Autodesk Inventor part; units mm, degrees
ref_plane "YZ Plane" through (0, 0, 0) normal (1, 0, 0) x (0, 1, 0)
ref_plane "XZ Plane" through (0, 0, 0) normal (0, 1, 0) x (-1, 0, 0)
ref_plane "XY Plane" through (0, 0, 0) normal (0, 0, 1) x (1, 0, 0)
sketch "Sketch1" plane through (0, 0, 0) normal (0, 1, 0) x (-1, 0, 0)
  circle A0 centre (0, 0) radius 5.5
  circle A1 centre (0, 0) radius 7
  dimension "d0" = 11
  dimension "d1" = 14
extrude "Extrusion1" add sketch "Sketch1" along normal blind 10
thread "Thread1"
sketch "Sketch2" plane through (0, 0, 0) normal (0, -1, 0) x (1, 0, 0)
  circle A0 centre (0, 5.4798) radius 0.75
  point P0 (0, 0)
  dimension "d6" = 1.5
extrude "Extrusion2" add sketch "Sketch2" against normal blind 10
sketch "Sketch3" plane through (0, 10, 0) normal (0, 1, 0) x (1, 0, 0)
  circle A0 centre (0, 0) radius 5.5
  circle A1 centre (0, 0) radius 12.5
  dimension "d9" = 11
  dimension "d10" = 25
extrude "Extrusion3" add sketch "Sketch3" along normal blind 1.5 contours A0 | A1
sketch "Sketch4" plane through (0, 11.5, 0) normal (0, 1, 0) x (1, 0, 0)
  line L0 (10.5, -6.0622) -> (0, -12.1244)
  line L1 (0, -12.1244) -> (-10.5, -6.0622)
  line L2 (-10.5, -6.0622) -> (-10.5, 6.0622)
  line L3 (-10.5, 6.0622) -> (0, 12.1244)
  line L4 (0, 12.1244) -> (10.5, 6.0622)
  line L5 (10.5, 6.0622) -> (10.5, -6.0622)
  circle A0 centre (0, 0) radius 7.5
  dimension "d14" = 15
extrude "Extrusion4" add sketch "Sketch4" along normal blind 4.5
sketch "Sketch5" plane through (0, 16, 0) normal (0, 1, 0) x (1, 0, 0)
  circle A0 centre (0, 0) radius 7.5
  circle A1 centre (0, 0) radius 9.5
  dimension "d17" = 15
  dimension "d18" = 19
extrude "Extrusion5" add sketch "Sketch5" along normal blind 6
thread "Thread2"
sketch "Sketch6" plane through (0, 22, 0) normal (0, 1, 0) x (1, 0, 0)
  line L0 (0.5, -8.4949) -> (-0.5, -8.4949)
  line L1 (-0.5, -8.4949) -> (-0.5, -6.4949)
  line L2 (-0.5, -6.4949) -> (0.5, -6.4949)
  line L3 (0.5, -6.4949) -> (0.5, -8.4949)
  line L4 (0.5, -8.4949) -> (-0.5, -6.4949) construction
  line L5 (-0.5, -8.4949) -> (0.5, -6.4949) construction
  line L6 (3.8144, 7.6068) -> (4.6804, 7.1068)
  line L7 (4.6804, 7.1068) -> (3.6804, 5.3747)
  line L8 (3.6804, 5.3747) -> (2.8144, 5.8747)
  line L9 (2.8144, 5.8747) -> (3.8144, 7.6068)
  line L10 (3.8144, 7.6068) -> (3.6804, 5.3747) construction
  line L11 (4.6804, 7.1068) -> (2.8144, 5.8747) construction
  line L12 (-4.6804, 7.1068) -> (-3.8144, 7.6068)
  line L13 (-3.8144, 7.6068) -> (-2.8144, 5.8747)
  line L14 (-2.8144, 5.8747) -> (-3.6804, 5.3747)
  line L15 (-3.6804, 5.3747) -> (-4.6804, 7.1068)
  line L16 (-4.6804, 7.1068) -> (-2.8144, 5.8747) construction
  line L17 (-3.8144, 7.6068) -> (-3.6804, 5.3747) construction
  point P0 (0, 0)
  point P1 (0, -7.4949)
  point P2 (0, 0)
  point P3 (3.7474, 6.4907)
  point P4 (-3.7474, 6.4907)
  dimension "d23" = 1
  dimension "d24" = 2
  dimension "d27" = 150
  dimension "d31" = 210
extrude "Extrusion6" add sketch "Sketch6" against normal blind 10.5
chamfer "Chamfer1" distance 1.5 angle 45 6 edges at (-10.5, 13.75, 6.0622) (-10.5, 13.75, -6.0622) (0, 13.75, 12.1244) (10.5, 13.75, 6.0622) (10.5, 13.75, -6.0622) (0, 13.75, -12.1244)
sketch "Sketch8" plane through (0, 0, 0) normal (0, 0, 1) x (1, 0, 0)
  line L0 (10.5, 16) -> (9.201, 16)
  line L1 (12.5, 11.5) -> (-12.5, 11.5)
  line L2 (10.5, 16) -> (12.5, 16)
  line L3 (12.5, 16) -> (12.5, 11.5)
  line L4 (12.5, 11.5) -> (10.5, 11.5)
  line L5 (10.5, 11.5) -> (10.5, 16)
  line L6 (-10.5, 16) -> (-10.5, 11.5)
  line L7 (-12.5, 11.5) -> (-10.5, 11.5)
  line L8 (-10.5, 11.5) -> (-10.5, 16)
  line L9 (-10.5, 16) -> (-12.5, 16)
  line L10 (-12.5, 16) -> (-12.5, 11.5)
  line L11 (-13, 11) -> (-10, 11)
  line L12 (-10, 11) -> (-10, 16.5)
  line L13 (-10, 16.5) -> (-13, 16.5)
  line L14 (-13, 16.5) -> (-13, 11)
  line L15 (12, 12) -> (12, 15.5)
  line L16 (12, 15.5) -> (11, 15.5)
  line L17 (11, 15.5) -> (11, 12)
  line L18 (11, 12) -> (12, 12)
  dimension "d43" = 0.5
  dimension "d44" = 0.5
extrude "Extrusion8" add sketch "Sketch8" along normal mid plane 0.5
properties part number "nut"
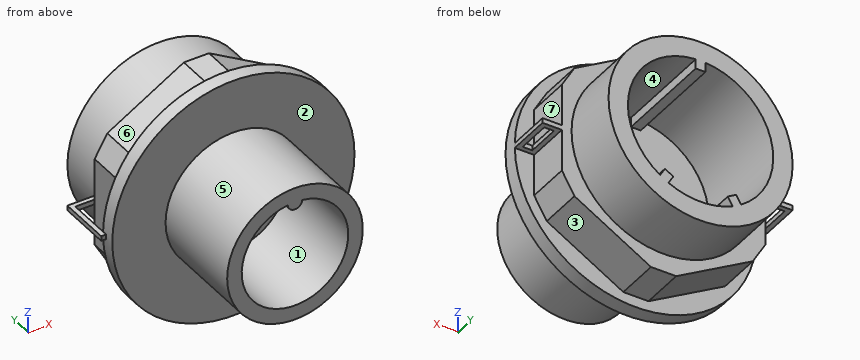
Geometry check sheet. Reference: the model listing, model coordinates, mm. Face numbers are marked on the shaded views. A direction names the side the tool comes from. Round coordinates to 2 decimals unless told otherwise and drop trailing zeros. Loops run counter-clockwise (first coordinate to the right, second up) from the corner with the lowest first, then second, coordinate; pieces in that order, holes last. Notation, with made-up numbers: (-27.75, 62) - (-20.75, 62) arc R32 ccw to (-20.75, 93) - close; hole circle Ø2 at (-12, 68.25). An arc over 180 degrees is marked (long way). Write item = value, one per line. Start each with the question number.
1. Section check C-C on x = 0. Enter the section's corners in (y, z), then the cut area to 3 significant figures.
2. Depth check by flat-ended pin: pin 1 (4 mm diameter, centred on x = 3.5, y = 12, fed in from +Z); pin 2 (2 mm diameter, centred on x = 2, z = -2, fed in from -Y); pin 3 (3.5 mm diameter, centred on y = 13.5, z = -3, fed in from +X). Enter the tip coordinate at first touch or a pass-through.
3. Section check D-D on z = 2. Enter the section's corners in (x, y).
4. Set-up check for the marked faces 5, 6 and 7: record each of +Z, -Z, +X, -X, +Y, -Y from which the full face is reachable in a straight line by a thin tool's end or side.
5. Mould release check, pull along X, two halves, no side actions. Record for the marked faces 1, 2, 3 and 4: released by +X, released by -X, zero draft, split by the parting line, or undercut.
6. Section check B-B on y = 17.25. Enter the section's corners in (x, z).
7. Section check A-A on y = 13. Give the number of separate pieces and of enclosed holes in the cut face, then the cut area to 3 significant figures.
8. Thickness scan on line 1 (Z direction, x = 0, y = 4); line 2 (Y direction, x = 6.25, z = 4); line 3 (Z direction, x = 2.75, y = 17.75). Record the ranges inside material, lowest first.
Working result:
q1.outline = (0, -7) - (10, -7) - (10, -12.5) - (11.5, -12.5) - (11.5, -11.37) - (16, -11.37) - (16, -9.5) - (22, -9.5) - (22, -7.5) - (11.5, -7.5) - (11.5, 6.49) - (22, 6.49) - (22, 9.5) - (16, 9.5) - (16, 11.37) - (11.5, 11.37) - (11.5, 12.5) - (10, 12.5) - (10, 7) - (0, 7) - (0, 4.73) - (10, 4.73) - (10, -5.5) - (0, -5.5) - close
q1.area = 145 mm^2
q2.pin_1 = 12.4
q2.pin_2 = 10
q2.pin_3 = 10.5
q3.outline = (-12.34, 10) - (-6.71, 10) - (-6.71, 0) - (-5.12, 0) - (-5.12, 10) - (5.12, 10) - (5.12, 0) - (6.71, 0) - (6.71, 10) - (12.34, 10) - (12.34, 11.5) - (10.5, 11.5) - (10.5, 16) - (9.29, 16) - (9.29, 22) - (7.23, 22) - (7.23, 11.5) - (-7.23, 11.5) - (-7.23, 22) - (-9.29, 22) - (-9.29, 16) - (-10.5, 16) - (-10.5, 11.5) - (-12.34, 11.5) - close
q4.face_5 = -Y
q4.face_6 = +Z, -X, +Y
q4.face_7 = +Z, +X, +Y
q5.face_1 = undercut
q5.face_2 = zero draft
q5.face_3 = released by +X
q5.face_4 = undercut
q6.outline = circle Ø19 at (0, 0); hole (-4.17, -6.23) - (-3.68, -5.37) - (-2.81, -5.87) - (-3.31, -6.73) arc R7.5 ccw to (3.31, -6.73) - (2.81, -5.87) - (3.68, -5.37) - (4.17, -6.23) arc R7.5 ccw to (0.5, 7.48) - (0.5, 6.49) - (-0.5, 6.49) - (-0.5, 7.48) arc R7.5 ccw to start
q7.separate_pieces = 3
q7.enclosed_holes = 1
q7.area = 203 mm^2
q8.line_1 = -7 to -5.5, 4.73 to 7
q8.line_2 = 10 to 11.5
q8.line_3 = -9.09 to -6.98, 6.98 to 9.09
